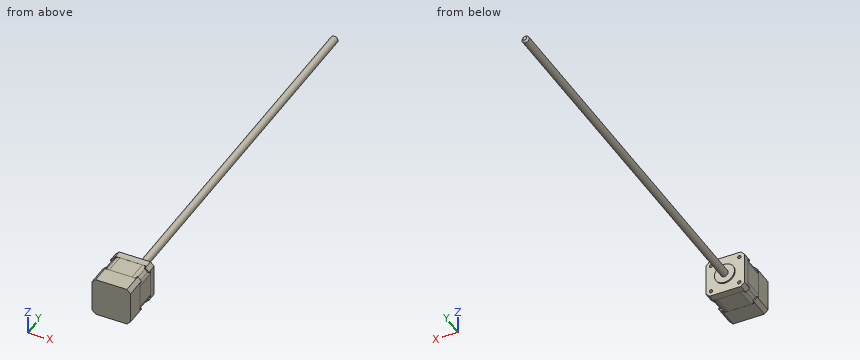
```python
from build123d import *

# Parameters (mm, degrees)
ESBO_O1_W              = 42.3
ESBO_O1_H              = 42.3
UPPERBODY_DEPTH        = 8
CHANFRO1_SIZE          = 4
ESBO_O2_R              = 11
ESBO_O2_R_2            = 4.1
LITTLETOPCIRCLE_DEPTH  = 1.5
ESBO_O3_R              = 1.853680608
MOUNTINGHOLES_DEPTH    = 25
PADR_OCIRCULAR1_COUNT  = 4
LITTLEMETALTABS_DEPTH  = 3
PADR_OCIRCULAR2_COUNT  = 4
MIDDLEBODY_DEPTH       = 22
FILETE1_R              = 6
ESBO_O9_W              = 42.3
ESBO_O9_H              = 42.3
BOTTOMBODY_DEPTH       = 8
CHANFRO5_SIZE          = 4
LITTLEMETALTABS2_DEPTH = 3
PADR_OCIRCULAR3_COUNT  = 4
ESBO_O4_R              = 4
LEADSCREW_DEPTH        = 425
CHANFRO2_SIZE          = 2
EXTRUDE_1_DEPTH        = 12


with BuildPart() as part:
    # Esbo_o1 → UpperBody (new body)
    with BuildSketch(Plane(origin=(0, 0, 0), x_dir=(1, 0, 0), z_dir=(0, 1, 0))):
        Rectangle(ESBO_O1_W, ESBO_O1_H)
    extrude(amount=UPPERBODY_DEPTH)

    # Chanfro1
    chanfro1_edges = [part.edges().sort_by_distance(p)[0] for p in [
        (21.15, 4, 21.15),
        (-21.15, 4, 21.15),
        (-21.15, 4, -21.15),
        (21.15, 4, -21.15),
    ]]
    chamfer(chanfro1_edges, length=CHANFRO1_SIZE)

    # Esbo_o2 → LittleTopCircle (add)
    with BuildSketch(Plane(origin=(0, 8, 0), x_dir=(1, 0, 0), z_dir=(0, 1, 0))):
        with Locations(Location((0, 0, 0), (0, 0, 270))):
            Circle(ESBO_O2_R)
        with Locations(Location((0, 0, 0), (0, 0, 270))):
            Circle(ESBO_O2_R_2, mode=Mode.SUBTRACT)
    extrude(amount=LITTLETOPCIRCLE_DEPTH)

    # Esbo_o3 → MountingHoles (cut)
    with BuildSketch(Plane(origin=(0, 8, 0), x_dir=(1, 0, 0), z_dir=(0, 1, 0))):
        with Locations(Location((-15.5, 15.5, 0), (0, 0, 270))):
            Circle(ESBO_O3_R)
    mountingholes = extrude(amount=-MOUNTINGHOLES_DEPTH, mode=Mode.SUBTRACT)

    # Padr_oCircular1: MountingHoles ×4 about axis
    padr_ocircular1_axis = Axis((0, 0, 0), (0, 1, 0))
    for i in range(1, PADR_OCIRCULAR1_COUNT):
        add(mountingholes.rotate(padr_ocircular1_axis, i * 360 / PADR_OCIRCULAR1_COUNT), mode=Mode.SUBTRACT)

    # Esbo_o7 → LittleMetalTabs (add)
    with BuildSketch(Plane.XZ):
        Polygon((-19.65, -16.528679656), (-21.15, -16.528679656), (-21.15, -17.15), (-17.15, -21.15), (-16.528679656, -21.15), (-16.528679656, -19.65), align=None)
    littlemetaltabs = extrude(amount=LITTLEMETALTABS_DEPTH)

    # Padr_oCircular2: LittleMetalTabs ×4 about axis
    padr_ocircular2_axis = Axis((0, 0, 0), (0, 1, 0))
    for i in range(1, PADR_OCIRCULAR2_COUNT):
        add(littlemetaltabs.rotate(padr_ocircular2_axis, i * 360 / PADR_OCIRCULAR2_COUNT))

    # Esbo_o8 → MiddleBody (add)
    with BuildSketch(Plane.XZ):
        Polygon((-14.9, 21.1), (14.9, 21.1), (21.1, 14.9), (21.1, -14.9), (14.9, -21.1), (-14.9, -21.1), (-21.1, -14.9), (-21.1, 14.9), align=None)
    extrude(amount=MIDDLEBODY_DEPTH)

    # Filete1
    filete1_edges = [part.edges().sort_by_distance(p)[0] for p in [
        (-21.1, -11, -14.9),
        (-14.9, -11, -21.1),
        (14.9, -11, -21.1),
        (21.1, -11, -14.9),
        (21.1, -11, 14.9),
        (14.9, -11, 21.1),
        (-14.9, -11, 21.1),
        (-21.1, -11, 14.9),
    ]]
    fillet(filete1_edges, radius=FILETE1_R)

    # Esbo_o9 → BottomBody (add)
    with BuildSketch(Plane.XZ.offset(22)):
        Rectangle(ESBO_O9_W, ESBO_O9_H)
    extrude(amount=BOTTOMBODY_DEPTH)

    # Chanfro5
    chanfro5_edges = [part.edges().sort_by_distance(p)[0] for p in [
        (21.15, -26, -21.15),
        (21.15, -26, 21.15),
        (-21.15, -26, 21.15),
        (-21.15, -26, -21.15),
    ]]
    chamfer(chanfro5_edges, length=CHANFRO5_SIZE)

    # Esbo_o10 → LittleMetalTabs2 (add)
    with BuildSketch(Plane(origin=(0, -22, 0), x_dir=(1, 0, 0), z_dir=(0, 1, 0))):
        Polygon((-16.528679656, -21.15), (-16.528679656, -19.65), (-19.65, -16.528679656), (-21.15, -16.528679656), (-21.15, -17.15), (-17.15, -21.15), align=None)
    littlemetaltabs2 = extrude(amount=LITTLEMETALTABS2_DEPTH)

    # Padr_oCircular3: LittleMetalTabs2 ×4 about axis
    padr_ocircular3_axis = Axis((0, 0, 0), (0, 1, 0))
    for i in range(1, PADR_OCIRCULAR3_COUNT):
        add(littlemetaltabs2.rotate(padr_ocircular3_axis, i * 360 / PADR_OCIRCULAR3_COUNT))

    # Esbo_o4 → LeadScrew (add)
    with BuildSketch(Plane(origin=(0, 8, 0), x_dir=(1, 0, 0), z_dir=(0, 1, 0))):
        with Locations(Location((0, 0, 0), (0, 0, 270))):
            Circle(ESBO_O4_R)
    extrude(amount=LEADSCREW_DEPTH)

    # Chanfro2
    chanfro2_edges = [part.edges().sort_by_distance(p)[0] for p in [
        (0, 433, -4),
    ]]
    chamfer(chanfro2_edges, length=CHANFRO2_SIZE)

    # Sketch 6 → Extrude 1 (add)
    with BuildSketch(Plane.XZ.offset(30)):
        Polygon((21.15, -17.15), (21.15, 17.15), (17.15, 21.15), (-17.15, 21.15), (-21.15, 17.15), (-21.15, -17.15), (-17.15, -21.15), (17.15, -21.15), align=None)
    extrude(amount=EXTRUDE_1_DEPTH)


solid = part.part
```
Source: CAD feature listing. Evaluate the final solid. Frame: model axes, mm. Give positions to 0.01 mm unless a question says otherwise; leave off trailing zeros. Loops run counter-clockwise (first coordinate to the right, second up) from the corner with the lowest first, then second, coordinate; pieces in that order, holes last. Notation, with made-up numbers: (59.5, 2.5) -> (71.5, 2.5) arc R27 cw to (71.5, 29.5) -> close; hole circle Ø8 at (33.25, 26). An arc over 180 degrees is marked (long way). Use a Markdown table: item, result. Add a question column.
(1) First-contact query: pin 1 Ø1.6 at (y, z) = (-1, 20) entering from +X; pin 2 Ø5 at (y, z) = (324.5, 8.5) entering from -X; pin 3 Ø4 at (x, z) = (2, -1.5) entering from +Y; pin 4 Ø6.5 at (y, z) = (-10.5, 1) entering from +X. Flat tips, straight axial feed; report the tip coordinate or a pass-through.
(2) Section query A-A (y = -10). Output: boundary loops of the cut face in (x, z), then the cut area to 3 significant figures.
(3) Ray query, line 1 (X direction, y = 4, z = -15); line 2 (X direction, y = 3.75, z = 15.5); line 3 (Y direction, x = 19, z = 8). Return the intervals inside material, ascending.
Checked values:
| question | item | result |
|---|---|---|
| 1 | pin 1 | x = 19.1 |
| 1 | pin 2 | through |
| 1 | pin 3 | y = 433 |
| 1 | pin 4 | x = 21.1 |
| 2 | outline | (-21.1, -12.41) arc R6 ccw to (-19.34, -16.66) -> (-16.66, -19.34) arc R6 ccw to (-12.41, -21.1) -> (12.41, -21.1) arc R6 ccw to (16.66, -19.34) -> (19.34, -16.66) arc R6 ccw to (21.1, -12.41) -> (21.1, 12.41) arc R6 ccw to (19.34, 16.66) -> (16.66, 19.34) arc R6 ccw to (12.41, 21.1) -> (-12.41, 21.1) arc R6 ccw to (-16.66, 19.34) -> (-19.34, 16.66) arc R6 ccw to (-21.1, 12.41) -> close |
| 2 | area | 1,700 mm^2 |
| 3 | line 1 | -21.15 to -17.28, -13.72 to 13.72, 17.28 to 21.15 |
| 3 | line 2 | -21.15 to -17.35, -13.65 to 13.65, 17.35 to 21.15 |
| 3 | line 3 | -42 to 8 |
